from build123d import *

# Parameters (mm, degrees)
F1_R     = 11
F2_DEPTH = 9
F3_SIZE  = 0.5
F4_SIZE  = 1


with BuildPart() as f2:
    # F1 (on Top) → F2 (new body)
    with BuildSketch(Plane.XY):
        with BuildLine():
            ThreePointArc((12.1243558114, 23.0000002745), (13.5229616091, 26.3765335216), (14, 30))
            ThreePointArc((14, 30), (-3.6234666891, 43.5229615526), (-12.1243555933, 22.9999998966))
            ThreePointArc((-12.1243555933, 22.9999998966), (2.181e-07, 16), (12.1243558114, 23.0000002745))
        make_face()
        with Locations((0, 30)):
            Circle(F1_R, mode=Mode.SUBTRACT)
        with BuildLine():
            ThreePointArc((39.9807621135, -15), (35.8802570426, -5.1005050558), (25.9807620921, -1))
            ThreePointArc((25.9807620921, -1), (13.8564063651, -8.0000001654), (13.8564066408, -22.0000003122))
            ThreePointArc((13.8564066408, -22.0000003122), (29.6042289191, -28.5229615214), (39.9807621135, -15))
        make_face()
        with Locations((25.9807621135, -15)):
            Circle(F1_R, mode=Mode.SUBTRACT)
        with BuildLine():
            ThreePointArc((-11.9807621135, -15), (-16.0812671769, -5.1005050634), (-25.9807621135, -1))
            ThreePointArc((-25.9807621135, -1), (-38.105117752, -22.0000000252), (-13.8564064315, -21.9999999496))
            ThreePointArc((-13.8564064315, -21.9999999496), (-12.457800538, -18.6234666034), (-11.9807621135, -15))
        make_face()
        with Locations((-25.9807621135, -15)):
            Circle(F1_R, mode=Mode.SUBTRACT)
        with BuildLine():
            ThreePointArc((-12.1243554957, 7.0000002723), (-17.9807619774, 1.1435936181), (-25.9807621135, -1))
            ThreePointArc((-25.9807621135, -1), (-16.0812671769, -5.1005050634), (-11.9807621135, -15))
            ThreePointArc((-11.9807621135, -15), (-12.457800538, -18.6234666034), (-13.8564064315, -21.9999999496))
            ThreePointArc((-13.8564064315, -21.9999999496), (-7.9999999748, -16.1435935249), (0, -14))
            ThreePointArc((0, -14), (-12.1243557316, -6.9999998638), (-12.1243554957, 7.0000002723))
        make_face()
        with BuildLine():
            ThreePointArc((25.9807620921, -1), (17.9807619484, 1.1435936348), (12.124355473, 7.0000003117))
            ThreePointArc((12.124355473, 7.0000003117), (13.5229615215, 3.6234668052), (14, 0))
            ThreePointArc((14, 0), (9.8994949366, -9.8994949366), (0, -14))
            ThreePointArc((0, -14), (8.0000001561, -16.1435936296), (13.8564066408, -22.0000003122))
            ThreePointArc((13.8564066408, -22.0000003122), (13.8564063651, -8.0000001654), (25.9807620921, -1))
        make_face()
        with BuildLine():
            ThreePointArc((12.1243558114, 23.0000002745), (2.181e-07, 16), (-12.1243555933, 22.9999998966))
            ThreePointArc((-12.1243555933, 22.9999998966), (-10.5259488775, 19.141104664), (-9.9807621135, 15))
            ThreePointArc((-9.9807621135, 15), (-10.5259488522, 10.8588954302), (-12.1243554957, 7.0000002723))
            ThreePointArc((-12.1243554957, 7.0000002723), (-2.27e-08, 14), (12.124355473, 7.0000003117))
            ThreePointArc((12.124355473, 7.0000003117), (9.9807621135, 15.0000003384), (12.1243558114, 23.0000002745))
        make_face()
        with BuildLine():
            ThreePointArc((14, 0), (13.5229615215, 3.6234668052), (12.124355473, 7.0000003117))
            ThreePointArc((12.124355473, 7.0000003117), (-2.27e-08, 14), (-12.1243554957, 7.0000002723))
            ThreePointArc((-12.1243554957, 7.0000002723), (-12.1243557316, -6.9999998638), (0, -14))
            ThreePointArc((0, -14), (9.8994949366, -9.8994949366), (14, 0))
        make_face()
        Circle(F1_R, mode=Mode.SUBTRACT)
    extrude(amount=F2_DEPTH)

    # F3
    f3_edges = [f2.edges().sort_by_distance(p)[0] for p in [
        (-36.980762, -15, 9),
        (-11, 0, 9),
        (-11, 30, 9),
        (14.980762, -15, 9),
        (-36.980762, -15, 0),
        (-11, 0, 0),
        (14.980762, -15, 0),
        (-11, 30, 0),
    ]]
    chamfer(f3_edges, length=F3_SIZE)

    # F4
    f4_edges = [f2.edges().sort_by_distance(p)[0] for p in [
        (-38.105118, -22, 9),
        (0, -14, 9),
        (-12.124356, 7, 9),
        (0, 44, 9),
        (12.124356, 7, 9),
        (38.105118, -22, 9),
        (0, -14, 0),
        (-38.105118, -22, 0),
        (-12.124356, 7, 0),
        (0, 44, 0),
        (12.124356, 7, 0),
        (38.105118, -22, 0),
    ]]
    chamfer(f4_edges, length=F4_SIZE)


solid = f2.part
The listing builds one solid part. Answer for the finished solid, in the listing's coordinates (mm). Coordinates: 2 decimals unless noted, no trailing zeros. Write each loop counter-clockwise with the first axis right and the second up, starting at its lowest first coordinate (ties: lowest second). Pieces come first, ordered by that corner, then holes. Notation, with made-up numbers: M 68,35 L 84,35 A10 cw 84,42 Z; hole C -14,-9 d1. An arc over 180 degrees is marked long. Put each result on its own line as item: value. Start each with the question number.
1. Flat-ended cylindrical pins translate along their axes: P1, Ø5, axis at y = -5.5, z = 2.5, coming from the -X side; P2, Ø4, axis at y = 16.5, z = 5.5, coming from the -X side. Find the tip coordinate at first contact, or state that the pin passes through.
2. Consider line 1 (Y direction, x = 0.5, z = 2.5); line 2 (X direction, y = -5.5, z = 3.5); line 3 (Y direction, x = 7, z = 5). Determine where each line is inside the solid, lowest interval first. Write a range as from..to.
3. A cutting plane is placed at B-B on y = -24.5. Count the separate pieces of the cut face and the enclosed holes in it, then the cut area to 3 significant figures.
4. A cutting plane is placed at A-A on z = 4. Write down the section's boundary in (x, y), then the cut area to 3 significant figures.
5. For a pull along Y with two mould halves and no side action, classify faces 1 (the cylindrical face through (-38.305, -21.642, 4.451)), 2 (the cylindrical face through (23.6, -25.74, 4.44)), 3 (the flat face through (-9, -8, 9)) as pulls with the +Y half, pulls with the -Y half, needs draft (parallel to the pull), parting line crosses it, or undercut.
Resolved:
1. P1: stops at x = -38.11
1. P2: stops at x = -10.37
2. line 1: y = -14.01..-10.99, 10.99..19.01, 40.99..43.99
2. line 2: x = -36.26..-31.53, -20.44..-9.53, 9.53..20.44, 31.53..36.26
2. line 3: y = -15.61..-8.49, 8.49..21.51, 38.49..42.12
3. separate pieces: 4
3. enclosed holes: 0
3. area: 163 mm2
4. outline: M -25.98,-1 A14 ccw long -13.86,-22 A16 cw 13.86,-22 A14 ccw long 25.98,-1 A16 cw 12.12,23 A14 ccw long -12.12,23 A16 cw Z; hole C -25.98,-15 d22; hole C 0,0 d22; hole C 0,30 d22; hole C 25.98,-15 d22
4. area: 1,240 mm2
5. face 1: parting line crosses it
5. face 2: undercut
5. face 3: needs draft
